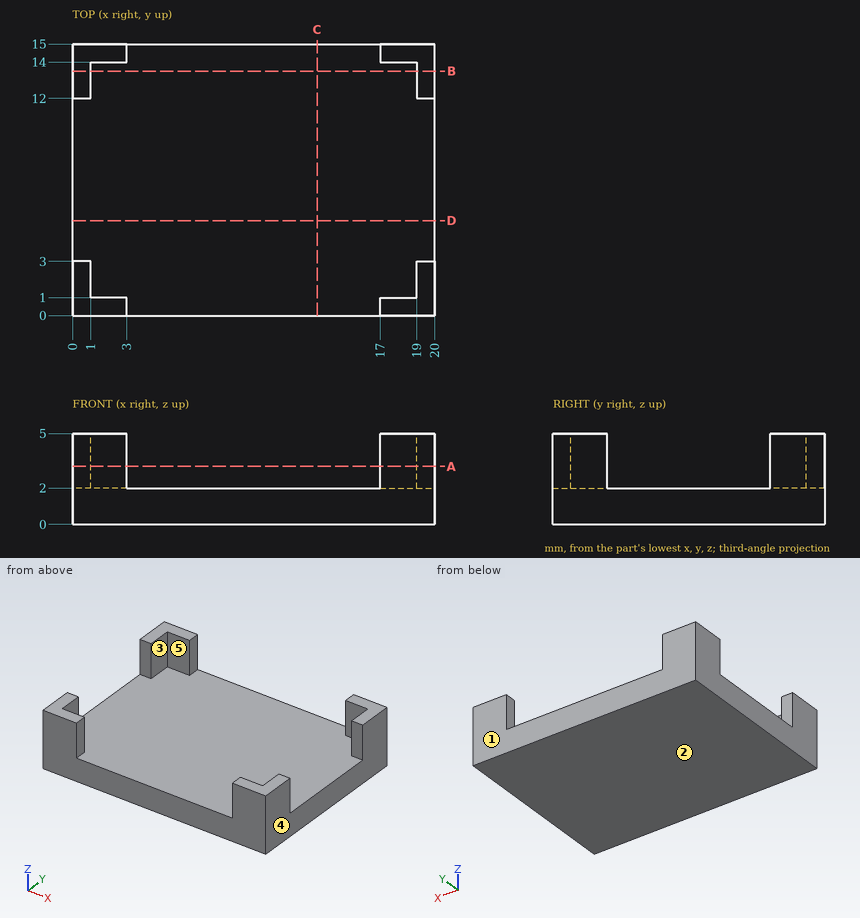
Part print with two shaded views. Sizes in mm from the minimum x, y, z corner. A direction names the side the tool comes from. Give positions to 0.01 mm unless a question says otherwise; leave off trailing zeros. Order: outer loops, then holes, each group sorted by start corner. A loop starts at its lowest first (then second) coordinate and runs counter-clockwise, first axis right, second up.
(1) Drill centre lines: L1, parallel to X at y = 2.5, z = 4.45; L2, parallel to Z at x = 1.5, y = 4.25. Where is each one in solid material? Low to high.
(2) Mould opens along Y. For the marked faces 1, 2 and 3 say: released by +Y, released by -Y, zero draft, split by the parting line, or undercut.
(3) Saw through at C-C, the plane x = 13.5. Give the cut face in (y, z), then the cut area to 3 significant figures.
(4) Tool access for the marked faces 4 and 5: list every direction of +Z, -Z, +X, -X, +Y, -Y with a clear straight run to the whole face (end or side of a thin tool).
(5) Saw through at B-B, the plane y = 13.5. Give the cut face in (x, z), then the cut area to 3 significant figures.
(6) Saw through at D-D, the plane y = 5.25. Give the cut face in (x, z), then the cut area to 3 significant figures.
(7) Saw through at A-A, the plane z = 3.2. Give the cut face in (x, y), then the cut area to 3 significant figures.
Results found:
1. L1: x = 0 to 1, 19 to 20
1. L2: z = 0 to 2
2. face 1: released by +Y
2. face 2: zero draft
2. face 3: undercut
3. outline: (0, 0) - (15, 0) - (15, 2) - (0, 2) - close
3. area: 30.0 mm2
4. face 4: +Z, -Z, +X, +Y, -Y
4. face 5: +Z
5. outline: (0, 0) - (20, 0) - (20, 5) - (19, 5) - (19, 2) - (1, 2) - (1, 5) - (0, 5) - close
5. area: 46.0 mm2
6. outline: (0, 0) - (20, 0) - (20, 2) - (0, 2) - close
6. area: 40.0 mm2
7. outline: (0, 0) - (3, 0) - (3, 1) - (1, 1) - (1, 3) - (0, 3) - close; (0, 12) - (1, 12) - (1, 14) - (3, 14) - (3, 15) - (0, 15) - close; (17, 0) - (20, 0) - (20, 3) - (19, 3) - (19, 1) - (17, 1) - close; (17, 14) - (19, 14) - (19, 12) - (20, 12) - (20, 15) - (17, 15) - close
7. area: 20.0 mm2
